The listing builds one solid part. Answer for the finished solid, in the listing's coordinates (mm). Coordinates: 2 decimals unless noted, no trailing zeros. Loops run counter-clockwise (first coordinate to the right, second up) from the corner with the lowest first, then second, coordinate; pieces in that order, holes last. Notation, with made-up numbers: M 61,60 L 105,60 A27 ccw 105,98 Z; hole C 11.5,7.5 d3. An arc over 180 degrees is marked long. Answer as a JSON object with one key per item and string values. Group by question number.
1. A cutting plane is placed at C-C on z = 8.75. Give the vertices of the cut face in (x, y).
2. Given pin 1 (1.5 mm diameter, centred on x = -5, z = 9, fed in from -Y); pin 2 (1.5 mm diameter, centred on x = -1.5, z = 3.5, fed in from +Y); pin 3 (5 mm diameter, centred on x = -1, y = -0.5, fed in from +Z); pin 4 (3 mm diameter, centred on x = 4, z = 8, fed in from +Y), each flat-ended and moving along its own axis, determine where each tip first touches the part or whether it passes through.
3. Determine the mould class of faces 1 (the face through (-0.1, -5.2, 1)), 2 (the face through (-0.867, 3.905, 5.423)), 3 (the face through (-1.08, 4.88, 5.68)) for opening direction Y: released by +Y, released by -Y, zero draft, split by the parting line, or undercut.
4. A cutting plane is placed at A-A on x = 0. Give the vertices of the cut face in (y, z), and give its area (4 significant figures).
5. Straight lines are drawn through the part: L1, parallel to Y at x = 0, z = 4.75; L2, parallel to Z at x = -7, y = -2.25; L3, parallel to Y at x = -1.75, z = 5.5. For each, find the intervals that lie inside material, in ascending order.
6. A cutting plane is placed at D-D on x = 6. Give the vertices of the cut face in (y, z), and give its area (3 significant figures).
Autodesk Inventor part; units mm, degrees
ref_plane "YZ Plane" through (0, 0, 0) normal (1, 0, 0) x (0, 1, 0)
ref_plane "XZ Plane" through (0, 0, 0) normal (0, 1, 0) x (-1, 0, 0)
ref_plane "XY Plane" through (0, 0, 0) normal (0, 0, 1) x (1, 0, 0)
sketch "スケッチ1" plane through (0, 0, 0) normal (0, 0, 1) x (1, 0, 0)
  circle A0 centre (0, 0) radius 4
  circle A1 centre (0, 0) radius 8
  dimension "d0" = 8
  dimension "d1" = 16
extrude "押し出し1" add sketch "スケッチ1" along normal blind 1
sketch "スケッチ2" plane through (0, 0, 1) normal (0, 0, 1) x (1, 0, 0)
  circle A0 centre (0, 0) radius 5
  circle A1 centre (0, 0) radius 8
  circle A2 centre (0, 0) radius 4
  dimension "d4" = 10
extrude "押し出し2" add sketch "スケッチ2" along normal blind 10 contours A0
chamfer "面取り1" distance 0.5 angle 45 1 edges at (-5, 0, 11)
properties part number "オイレスw10f8-10a" material "アセタール樹脂、黒"
From the geometry:
{
 "1": {"outline": "C 0,0 d10; hole C 0,0 d8"},
 "2": {"pin 1": "stops at y = -2.63", "pin 2": "stops at y = 4.94", "pin 3": "passes through", "pin 4": "stops at y = 4.33"},
 "3": {"face 1": "zero draft", "face 2": "undercut", "face 3": "split by the parting line"},
 "4": {"outline": "M -8,0 L -4,0 L -4,11 L -4.5,11 L -5,10.5 L -5,1 L -8,1 Z; M 4,0 L 8,0 L 8,1 L 5,1 L 5,10.5 L 4.5,11 L 4,11 Z", "area": "27.75 mm²"},
 "5": {"L1": "y = -5 to -4, 4 to 5", "L2": "z = 0 to 1", "L3": "y = -4.68 to -3.6, 3.6 to 4.68"},
 "6": {"outline": "M -5.29,0 L 5.29,0 L 5.29,1 L -5.29,1 Z", "area": "10.6 mm²"}
}
